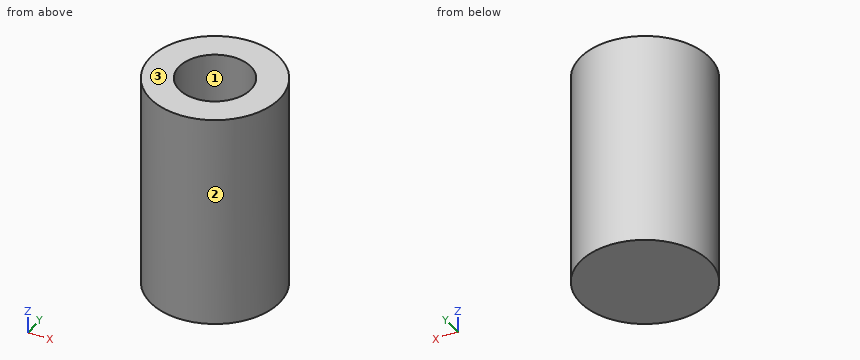
Autodesk Fusion 360 part; units mm, degrees
sketch "Sketch1" plane through (0, 0, 0) normal (0, 0, 1) x (1, 0, 0)
  circle A0 centre (25, 25) radius 2.5
  circle A1 centre (25, 25) radius 4.5
  dimension "d1" = 5
  dimension "d2" = 9
extrude "Extrude1" add sketch "Sketch1" along normal blind 10 contours A0 | A1
sketch "Sketch2" plane through (0, 0, 10) normal (0, 0, 1) x (-1, 0, 0)
  circle A0 centre (-25, -25) radius 4.5
extrude "Extrude2" add sketch "Sketch2" along normal blind 5
sketch "Sketch3" plane through (0, 0, 15) normal (0, 0, 1) x (-1, 0, 0)
  circle A0 centre (-25, -25) radius 4.5
  circle A1 centre (-25, -25) radius 2.5
  dimension "d7" = 5
extrude "Extrude3" cut sketch "Sketch3" against normal blind 12 contours A1
Geometry: final body of the model. Coordinates: model frame, mm. Face numbers are marked on the shaded views. Round coordinates to 2 decimals unless told otherwise and drop trailing zeros. Loops run counter-clockwise (first coordinate to the right, second up) from the corner with the lowest first, then second, coordinate; pieces in that order, holes last. Notation, with made-up numbers: (35, 28.5) -> (80, 28.5) arc R35 ccw to (80, 60.5) -> close; hole circle Ø6 at (-28, 80.5). An arc over 180 degrees is marked (long way). Use one line per item in the form item = value. Start each with the question number.
1) Section C-C on z = 4.75. Output: boundary loops of the cut face in (x, y).
2) Section D-D on z = 1. Output: boundary loops of the cut face in (x, y).
3) Draft query along X for the marked faces 1, 2 and 3. Return one class per face: released by +X, released by -X, zero draft, split by the parting line, or undercut.
4) First-contact query: P1, Ø3, axis at x = 25, y = 25, coming from the +Z side; P2, Ø1.5, axis at y = 27, z = 10.5, coming from the +X side; P3, Ø1.5, axis at x = 27.5, z = 9, coming from the +Y side. Flat tips, straight axial feed; report the tip coordinate or a pass-through.
5) Section A-A on x = 25. Output: boundary loops of the cut face in (y, z), then the cut area to 3 significant figures.
6) Line query: L1, parallel to Y at x = 25, z = 8.5; L2, parallel to Z at x = 23.5, y = 26.25. Output: solid intervals per line, ascending.
Response:
q1.outline = circle Ø9 at (25, 25); hole circle Ø5 at (25, 25)
q2.outline = circle Ø9 at (25, 25)
q3.face_1 = undercut
q3.face_2 = split by the parting line
q3.face_3 = zero draft
q4.P1 = 3
q4.P2 = 29.32
q4.P3 = 29.15
q5.outline = (20.5, 0) -> (29.5, 0) -> (29.5, 15) -> (27.5, 15) -> (27.5, 3) -> (22.5, 3) -> (22.5, 15) -> (20.5, 15) -> close
q5.area = 75.0 mm^2
q6.L1 = 20.5 to 22.5, 27.5 to 29.5
q6.L2 = 0 to 3
